Could you check a few things on this drawing? It's one solid part, dimensions in mm from its lowest x, y, z. Give positions to 0.01 mm unless a question says otherwise; leave off trailing zeros. Order: outer loops, then holes, each group sorted by start corner. A loop starts at its lowest first (then second) coordinate and runs counter-clockwise, first axis right, second up. Notation, with made-up numbers: (-15, 44.25) - (24, 44.25) arc R18 ccw to (24, 69.25) - close; hole circle Ø2 at (81.5, 72). An arc over 180 degrees is marked (long way). One line per question, with ' | ' between items. Start each with the question number.
1. Imagine slicing it at B-B (x = 10). Please give me the cut outline in (y, z), and give its area (3 significant figures).
2. I need wall thicknesses on probe 1 along Y at (x, z) = (110, 1); probe 2 along X at (y, z) = (9.5, 2.1). Which ranges of each line are inside material? Lowest first, please. Write a range as from..to.
3. Imagine slicing it at A-A (y = 10). Please give me the cut outline in (x, z).
4. Imagine slicing it at C-C (z = 1.25). Please give me the cut outline in (x, y).
5. For P1, Ø3.5, axis at x = 10, y = 10, coming from the -Z side, with a flat end and sliding along its axis, tell me the tip position at first contact or that it passes through.
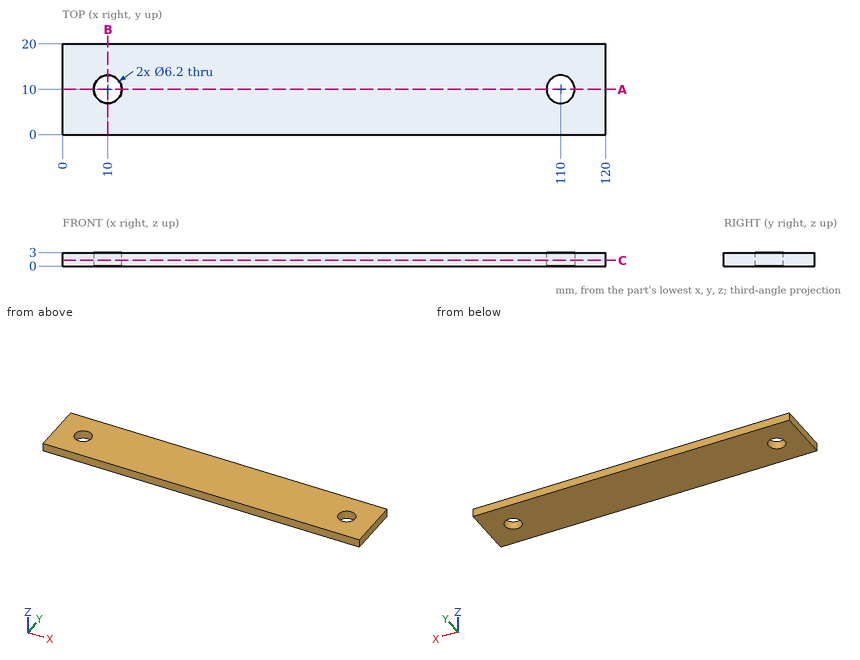
Results found:
1) outline: (0, 0) - (6.9, 0) - (6.9, 3) - (0, 3) - close; (13.1, 0) - (20, 0) - (20, 3) - (13.1, 3) - close | area: 41.4 mm2
2) probe 1: y = 0..6.9, 13.1..20 | probe 2: x = 0..6.94, 13.06..106.94, 113.06..120
3) outline: (0, 0) - (6.9, 0) - (6.9, 3) - (0, 3) - close; (13.1, 0) - (106.9, 0) - (106.9, 3) - (13.1, 3) - close; (113.1, 0) - (120, 0) - (120, 3) - (113.1, 3) - close
4) outline: (0, 0) - (120, 0) - (120, 20) - (0, 20) - close; hole circle Ø6.2 at (10, 10); hole circle Ø6.2 at (110, 10)
5) P1: passes through
